from build123d import *

# Parameters (mm, degrees)
SKETCH_W     = 21.75
SKETCH_H     = 6.75
PAD_DEPTH    = 13
SKETCH001_W  = 4
SKETCH001_H  = 4
POCKET_DEPTH = 10
CHAMFER_SIZE = 1


with BuildPart() as part:
    # Sketch → Pad (new body)
    with BuildSketch(Plane.XY):
        Rectangle(SKETCH_W, SKETCH_H)
    extrude(amount=PAD_DEPTH)

    # Sketch001 (on Face6 of Pad) → Pocket (cut)
    with BuildSketch(Plane.XY.offset(13)):
        Rectangle(SKETCH001_W, SKETCH001_H)
    extrude(amount=-POCKET_DEPTH, mode=Mode.SUBTRACT)

    # Chamfer
    chamfer_edges = [part.edges().sort_by_distance(p)[0] for p in [
        (0, 3.375, 0),
        (10.875, 0, 0),
        (0, -3.375, 0),
        (-10.875, 0, 0),
    ]]
    chamfer(chamfer_edges, length=CHAMFER_SIZE)


solid = part.part
The model under review builds one solid part; all positions refer to its coordinate system, in mm. A direction names the side the tool comes from. Round coordinates to 2 decimals unless told otherwise and drop trailing zeros. Loops run counter-clockwise (first coordinate to the right, second up) from the corner with the lowest first, then second, coordinate; pieces in that order, holes last. Notation, with made-up numbers: (65, 85) -> (104, 85) arc R12 cw to (104, 92) -> close; hole circle Ø9 at (7.25, 19). An arc over 180 degrees is marked (long way). Write item = value, one per line. Start each with the question number.
Item 1: Insertion check: pin 1 (2 mm diameter, centred on x = 0, y = 0.5, fed in from +Z). The pin has a flat end and moves straight along its axis. Give the tip position at first contact, or say it passes through.
Item 2: Take a section at B-B on x = -0.75. Give the boundary of the cut face in (y, z) (3 decimals), plus the area to 4 significant figures.
Item 3: Mouldability with a two-part tool opening along X and no side actions: class faces 1 (the flat face through (0, 0, 3)), 2 (the flat face through (-0.2, 2.3, 13)), 3 (the flat face through (10.875, 0, 7)) as released by +X, released by -X, zero draft, split by the parting line, or undercut.
Item 4: To check wall thickness, follow L1, parallel to X at y = 0, z = 4.25 (3 decimals); L2, parallel to Z at x = -0.75, y = -0.75; L3, parallel to Z at x = 3.25, y = -2.75 (3 decimals). State the ranges of each line that lie inside material, in increasing order.
Item 5: For faces 4 (the flat face through (-2, 0, 8)), 5 (the flat face through (-0.152, 2.868, 0.493)), list the 3-axis set-ups (+Z, -Z, +X, -X, +Y, -Y) from which the entire face can be reached by the end or side of a thin tool; tool diameter is ignored.
Item 6: Take a section at A-A on z = 8.75. Give the boundary of the cut face in (x, y) (3 decimals), plus the area to 3 significant figures.
Item 7: Take a section at C-C on y = 0. Give the boundary of the cut face in (x, z) (3 decimals).
Result:
q1.pin_1 = 3
q2.outline = (-3.375, 1) -> (-2.375, 0) -> (2.375, 0) -> (3.375, 1) -> (3.375, 13) -> (2, 13) -> (2, 3) -> (-2, 3) -> (-2, 13) -> (-3.375, 13) -> close
q2.area = 46.75 mm²
q3.face_1 = undercut
q3.face_2 = zero draft
q3.face_3 = released by +X
q4.L1 = -10.875 to -2, 2 to 10.875
q4.L2 = 0 to 3
q4.L3 = 0.375 to 13
q5.face_4 = +Z
q5.face_5 = -Z, +X, -X, +Y
q6.outline = (-10.875, -3.375) -> (10.875, -3.375) -> (10.875, 3.375) -> (-10.875, 3.375) -> close; hole (-2, -2) -> (2, -2) -> (2, 2) -> (-2, 2) -> close
q6.area = 131 mm²
q7.outline = (-10.875, 1) -> (-9.875, 0) -> (9.875, 0) -> (10.875, 1) -> (10.875, 13) -> (2, 13) -> (2, 3) -> (-2, 3) -> (-2, 13) -> (-10.875, 13) -> close
